For this review, take the finished solid that the model builds, in its own axes (mm). A direction names the side the tool comes from. Coordinates: 2 decimals unless noted, no trailing zeros. Loops run counter-clockwise (first coordinate to the right, second up) from the corner with the lowest first, then second, coordinate; pieces in that order, holes last. Notation, with made-up numbers: (18.5, 26) - (39.5, 26) arc R28 ccw to (39.5, 55) - close; hole circle Ø6 at (-35, -5). An arc over 180 degrees is marked (long way). One line per item, written item: value. Start each with the question number.
1. For faces 4 (the face through (16.4, 0.3, 12.7)), 5 (the face through (27.83, 5.64, 6.26)), list the 3-axis set-ups (+Z, -Z, +X, -X, +Y, -Y) from which the entire face can be reached by the end or side of a thin tool; tool diameter is ignored.
2. Take a section at C-C, the plane y = -13. State the section outline as (x, z) points, and give its area (3 significant figures).
3. Take a section at B-B, the plane z = 10. State the section outline as (x, y) points.
4. Take a section at A-A, the plane x = 28. State the section outline as (y, z) points.
5. Take a section at D-D, the plane y = 2.5. State the section outline as (x, z) points, and give its area (3 significant figures).
6. To check wall thickness, follow line 1 (X direction, y = -9, z = 6); line 2 (X direction, y = 4, z = 8); line 3 (Y direction, x = 0, z = 9.75). State the ranges of each line that lie inside material, in increasing order. Write a range as from..to.
7. The part is to be moulded in two halves that separate along Y. For faces 1 (the face through (-1, 19.05, 6)), 2 (the face through (-27.83, -5.64, 6.26)), 3 (the face through (-1, -19.05, 6)), say which applies: released by +Y, released by -Y, zero draft, split by the parting line, or undercut.
```python
from build123d import *

# Parameters (mm, degrees)
F0_W     = 76.2
F0_H     = 38.1
F1_DEPTH = 12.7


with BuildPart() as f1:
    # F0 (on Top) → F1 (new body)
    with BuildSketch(Plane.XY):
        Rectangle(F0_W, F0_H)
        Polygon((0, -18.530461), (-16.04785, -9.265231), (-16.04785, 9.265231), (0, 18.530461), (16.04785, 9.265231), (16.04785, -9.265231), align=None, mode=Mode.SUBTRACT)
        Polygon((-37.597824, 0), (-18.340401, 11.118278), (-18.340401, -11.118278), align=None, mode=Mode.SUBTRACT)
        Polygon((37.597822, 0), (18.340405, -11.118275), (18.340405, 11.118275), align=None, mode=Mode.SUBTRACT)
    extrude(amount=F1_DEPTH)


solid = f1.part
```
Solutions:
1. face 4: +Z, +X, -X, +Y, -Y
1. face 5: +Z, -Z
2. outline: (-38.1, 0) - (-9.58, 0) - (-9.58, 12.7) - (-38.1, 12.7) - close; (9.58, 0) - (38.1, 0) - (38.1, 12.7) - (9.58, 12.7) - close
2. area: 724 mm2
3. outline: (-38.1, -19.05) - (38.1, -19.05) - (38.1, 19.05) - (-38.1, 19.05) - close; hole (-37.6, 0) - (-18.34, -11.12) - (-18.34, 11.12) - close; hole (-16.05, -9.27) - (0, -18.53) - (16.05, -9.27) - (16.05, 9.27) - (0, 18.53) - (-16.05, 9.27) - close; hole (18.34, -11.12) - (37.6, 0) - (18.34, 11.12) - close
4. outline: (-19.05, 0) - (-5.54, 0) - (-5.54, 12.7) - (-19.05, 12.7) - close; (5.54, 0) - (19.05, 0) - (19.05, 12.7) - (5.54, 12.7) - close
5. outline: (-38.1, 0) - (-33.27, 0) - (-33.27, 12.7) - (-38.1, 12.7) - close; (-18.34, 0) - (-16.05, 0) - (-16.05, 12.7) - (-18.34, 12.7) - close; (16.05, 0) - (18.34, 0) - (18.34, 12.7) - (16.05, 12.7) - close; (33.27, 0) - (38.1, 0) - (38.1, 12.7) - (33.27, 12.7) - close
5. area: 181 mm2
6. line 1: -38.1..-22.01, -18.34..-16.05, 16.05..18.34, 22.01..38.1
6. line 2: -38.1..-30.67, -18.34..-16.05, 16.05..18.34, 30.67..38.1
6. line 3: -19.05..-18.53, 18.53..19.05
7. face 1: released by +Y
7. face 2: undercut
7. face 3: released by -Y
